Job drawing, mm, ordinate dimensions from the low corner. One solid piece. Round coordinates to 2 decimals unless told otherwise and drop trailing zeros. Write each loop counter-clockwise with the first axis right and the second up, starting at its lowest first coordinate (ties: lowest second). Pieces come first, ordered by that corner, then holes. Notation, with made-up numbers: (34, -33) - (77, -33) arc R31 ccw to (77, -4) - close; hole circle Ø8 at (-2, -2). An arc over 180 degrees is marked (long way). Write each question's results on one line, items separated by ' | '.
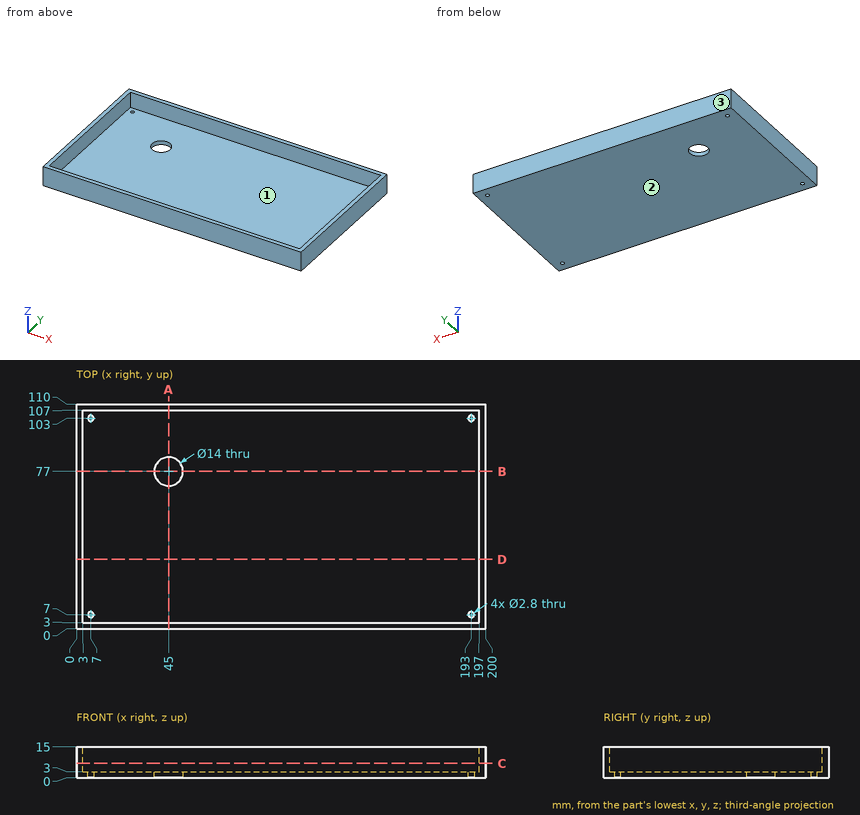
(1) Slice it at A-A, the plane x = 45. Write the cut outline in (y, z).
Worked answers:
outline: (0, 0) - (70, 0) - (70, 3) - (3, 3) - (3, 15) - (0, 15) - close; (84, 0) - (110, 0) - (110, 15) - (107, 15) - (107, 3) - (84, 3) - close
(2) Slice it at D-D, the plane y = 34. Write the cut outline in (x, z), and give its area (3 significant figures).
Worked answers:
outline: (0, 0) - (200, 0) - (200, 15) - (197, 15) - (197, 3) - (3, 3) - (3, 15) - (0, 15) - close | area: 672 mm2
(3) Slice it at C-C, the plane z = 7. Write the cut outline in (x, y), and give its area (3 significant figures).
Worked answers:
outline: (0, 0) - (200, 0) - (200, 110) - (0, 110) - close; hole (3, 3) - (197, 3) - (197, 107) - (3, 107) - close | area: 1,820 mm2
(4) Slice it at B-B, the plane y = 77. Write the cut outline in (x, z), and give its area (3 significant figures).
Worked answers:
outline: (0, 0) - (38, 0) - (38, 3) - (3, 3) - (3, 15) - (0, 15) - close; (52, 0) - (200, 0) - (200, 15) - (197, 15) - (197, 3) - (52, 3) - close | area: 630 mm2
(5) Drill centre lines: probe 1 along Y at (x, z) = (193, 0.6); probe 2 along X at (y, z) = (7, 0.95); probe 3 along Y at (x, z) = (65.5, 9). Where is each one in solid material? Low to high. Write a range as [from, to].
Worked answers:
probe 1: y = [0, 5.6], [8.4, 101.6], [104.4, 110] | probe 2: x = [0, 5.6], [8.4, 191.6], [194.4, 200] | probe 3: y = [0, 3], [107, 110]
(6) Flat gauge pin, fed straight in: pin 1 Ø2 at (x, y) = (178, 26.5) entering from +Z. Where does the tip first touch, or does it go through?
Worked answers:
pin 1: stops at z = 3
(7) Two-plate mould, pull along Y, no slides. Class the marked faces 1, 2 and 3: released by +Y, released by -Y, zero draft, split by the parting line, or undercut.
Worked answers:
face 1: undercut | face 2: zero draft | face 3: released by +Y
